Verification items for the finished model (mm, model axes). Face numbers are marked on the shaded views. A direction names the side the tool comes from. Give positions to 0.01 mm unless a question says otherwise; leave off trailing zeros. Write each loop counter-clockwise with the first axis right and the second up, starting at its lowest first coordinate (ties: lowest second). Pieces come first, ordered by that corner, then holes.
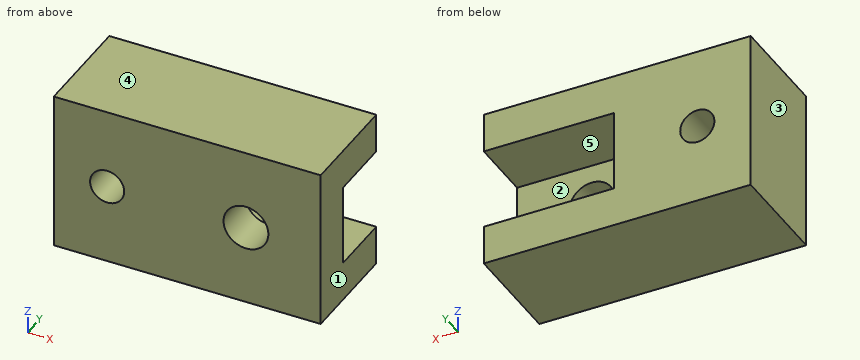
from build123d import *

# Parameters (mm, degrees)
SKETCH1_W           = 50
SKETCH1_H           = 30
BOSS_EXTRUDE1_DEPTH = 20
SKETCH3_W           = 15.2
SKETCH3_H           = 12
CUT_EXTRUDE1_DEPTH  = 51
SKETCH5_R           = 4.2
SKETCH5_R_2         = 3.2
CUT_EXTRUDE2_DEPTH  = 9
SKETCH6_W           = 25.6
SKETCH6_H           = 15.2
SKETCH6_R           = 3.2
BOSS_EXTRUDE2_DEPTH = 12


with BuildPart() as part:
    # Sketch1 → Boss-Extrude1 (new body)
    with BuildSketch(Plane(origin=(0, 0, 0), x_dir=(1, 0, 0), z_dir=(0, 1, 0))):
        Rectangle(SKETCH1_W, SKETCH1_H)
    extrude(amount=BOSS_EXTRUDE1_DEPTH)

    # Sketch3 → Cut-Extrude1 (cut, through all)
    with BuildSketch(Plane.ZY.offset(25)):
        with Locations((0, 14)):
            Rectangle(SKETCH3_W, SKETCH3_H)
    extrude(amount=-CUT_EXTRUDE1_DEPTH, mode=Mode.SUBTRACT)

    # Sketch5 → Cut-Extrude2 (cut, through all)
    with BuildSketch(Plane(origin=(0, 8, 0), x_dir=(1, 0, 0), z_dir=(0, 1, 0))):
        with Locations((11, 0)):
            Circle(SKETCH5_R)
        with Locations((-15, 0)):
            Circle(SKETCH5_R_2)
    extrude(amount=-CUT_EXTRUDE2_DEPTH, mode=Mode.SUBTRACT)

    # Sketch6 → Boss-Extrude2 (add)
    with BuildSketch(Plane(origin=(0, 8, 0), x_dir=(1, 0, 0), z_dir=(0, 1, 0))):
        with Locations((-12.2, 0)):
            Rectangle(SKETCH6_W, SKETCH6_H)
        with Locations((-15, 0)):
            Circle(SKETCH6_R, mode=Mode.SUBTRACT)
    extrude(amount=BOSS_EXTRUDE2_DEPTH)


solid = part.part
Item 1: Sectioned sample at D-D on x = 18.5. Record the cut outline in (y, z), then the cut area to 3 significant figures.
Answer key:
outline: (0, -15) - (20, -15) - (20, -7.6) - (8, -7.6) - (8, 7.6) - (20, 7.6) - (20, 15) - (0, 15) - close
area: 418 mm2
Item 2: Sectioned sample at B-B on z = 0. Record the cut outline in (x, y).
Answer key:
outline: (-25, 0) - (-18.2, 0) - (-18.2, 20) - (-25, 20) - close; (-11.8, 0) - (6.8, 0) - (6.8, 8) - (0.6, 8) - (0.6, 20) - (-11.8, 20) - close; (15.2, 0) - (25, 0) - (25, 8) - (15.2, 8) - close
Item 3: Sectioned sample at C-C on y = 8.5. Record the cut outline in (x, z).
Answer key:
outline: (-25, -15) - (25, -15) - (25, -7.6) - (0.6, -7.6) - (0.6, 7.6) - (25, 7.6) - (25, 15) - (-25, 15) - close; hole circle Ø6.4 at (-15, 0)
Item 4: Scan lines: line 1 along X through (y, z) = (4, 0); line 2 along Z through (x, y) = (-15, 6.5); line 3 along X through (y, z) = (18, -4). Record each from-to range of solid material in increasing order.
Answer key:
line 1: x = -25 to -18.2, -11.8 to 6.8, 15.2 to 25
line 2: z = -15 to -3.2, 3.2 to 15
line 3: x = -25 to 0.6
Item 5: Set-up check for the marked faces 1 and 2: record each of +Z, -Z, +X, -X, +Y, -Y from which the full face is reachable in a straight line by a thin tool's end or side.
Answer key:
face 1: +Z, -Z, +X, +Y, -Y
face 2: +X, +Y
Item 6: Sectioned sample at A-A on x = -15. Record the cut outline in (y, z), then the cut area to 3 significant figures.
Answer key:
outline: (0, -15) - (20, -15) - (20, -3.2) - (0, -3.2) - close; (0, 3.2) - (20, 3.2) - (20, 15) - (0, 15) - close
area: 472 mm2
Item 7: Depth check by flat-ended pin: pin 1 (3.5 mm diameter, centred on y = 14, z = -1.5, fed in from +X); pin 2 (1.5 mm diameter, centred on x = 2, z = -1, fed in from +Y). Enter the tip coordinate at first touch or a pass-through.
Answer key:
pin 1: stops at x = 0.6
pin 2: stops at y = 8
Item 8: Release check for a two-part mould opening along Z. For the marked faces 3, 4 and 5 record: released by +Z, released by -Z, zero draft, split by the parting line, or undercut.
Answer key:
face 3: zero draft
face 4: released by +Z
face 5: undercut
